Work out the finished part from the listing and answer in its coordinate system (mm). Give positions to 0.01 mm unless a question says otherwise; leave off trailing zeros. Order: outer loops, then holes, each group sorted by start corner. A loop starts at its lowest first (then second) coordinate and runs counter-clockwise, first axis right, second up. Notation, with made-up numbers: M -26,47 L -13,47 A24 ccw -13,66 Z; hole C 61,50 d9. An arc over 180 degrees is marked long. One line per item, written item: value.
Autodesk Inventor part; units mm, degrees
ref_plane "YZ Plane" through (0, 0, 0) normal (1, 0, 0) x (0, 1, 0)
ref_plane "XZ Plane" through (0, 0, 0) normal (0, 1, 0) x (-1, 0, 0)
ref_plane "XY Plane" through (0, 0, 0) normal (0, 0, 1) x (1, 0, 0)
sketch "Sketch1" plane through (0, 0, 0) normal (0, 0, 1) x (1, 0, 0)
  circle A0 centre (0, 0) radius 8.75
  circle A1 centre (0.25, 0) radius 24.8
  circle A2 centre (0.25, 0) radius 4.7
  circle A3 centre (-7.45, 0) radius 1.3
  circle A4 centre (-5.1947, -5.4447) radius 1.3
  circle A5 centre (0.25, -7.7) radius 1.3
  circle A6 centre (5.6947, -5.4447) radius 1.3
  circle A7 centre (7.95, 0) radius 1.3
  circle A8 centre (5.6947, 5.4447) radius 1.3
  circle A9 centre (0.25, 7.7) radius 1.3
  circle A10 centre (-5.1947, 5.4447) radius 1.3
  dimension "d0" = 17.5
  dimension "d1" = 49.6
  dimension "d3" = 9.4
  dimension "d4" = 2.6
  dimension "d7" = 360
extrude "Extrusion1" add sketch "Sketch1" along normal blind 2.5 contours A0 A7 | A0 A7 | A3 | A7 A0 A6 A5 A4 A10 A9 A8 | A8 A0 | A0 A8 | A6 A0 | A0 A6 | A9 A0 | A0 A9 | A5 A0 | A0 A5 | A10 A0 | A0 A10 | A4 A0 | A0 A4
properties part number "BigGearCenterer"
(1) Section A-A, the plane x = 0.25 is taken. Give the vertices of the cut face in (y, z), then the cut area to 3 significant figures.
Findings:
outline: M -9,0 L -4.7,0 L -4.7,2.5 L -9,2.5 Z; M 4.7,0 L 9,0 L 9,2.5 L 4.7,2.5 Z
area: 21.5 mm^2
(2) Determine the mould class of faces 1 (the cylindrical face through (-0.77, 4.59, 1.23)), 2 (the cylindrical face through (8.122, -3.255, 1.232)), 3 (the flat face through (-4, 4, 2.5)), 4 (the cylindrical face through (-3.249, -8.125, 1.232)) for opening direction X: pulls with the +X half, pulls with the -X half, needs draft (parallel to the pull), parting line crosses it, or undercut.
Findings:
face 1: undercut
face 2: pulls with the +X half
face 3: needs draft
face 4: pulls with the -X half
(3) Section D-D, the plane y = 5.5 is taken. Give the vertices of the cut face in (x, z).
Findings:
outline: M -6.81,0 L 6.99,0 L 6.99,2.5 L -6.81,2.5 Z
(4) Given P1, Ø1, axis at x = 6.5, z = 0.5, coming from the +Y side; P2, Ø1, axis at x = -2.5, y = 1.5, coming from the +Z side, each flat-ended and moving along its own axis, determine where each tip first touches the part or whether it passes through.
Findings:
P1: stops at y = 6.71
P2: passes through
(5) Find the intervals of material crossed by probe 1 along Y at (x, z) = (0.25, 1.5); probe 2 along Y at (x, z) = (-2.5, 1.7); probe 3 along X at (y, z) = (2, 0.55), in increasing order. Write a range as from..to.
Findings:
probe 1: y = -9..-4.7, 4.7..9
probe 2: y = -8.39..-3.81, 3.81..8.39
probe 3: x = -8.52..-4, 4.5..8.52
(6) Section B-B, the plane z = 0.6 is taken. Give the vertices of the cut face in (x, y), then the cut area to 3 significant figures.
Findings:
outline: M -6.37,-6 A1.3 ccw -5.69,-6.65 A8.75 ccw -0.54,-8.73 A1.3 ccw 1.1,-8.68 A8.75 ccw 5.58,-6.74 A1.3 ccw 6.98,-5.27 A8.75 ccw 8.68,-1.07 A1.3 ccw 8.68,1.07 A8.75 ccw 6.98,5.27 A1.3 ccw 5.58,6.74 A8.75 ccw 1.1,8.68 A1.3 ccw -0.54,8.73 A8.75 ccw -5.69,6.65 A1.3 ccw -6.37,6 A8.75 ccw Z; hole C 0.25,0 d9.4
area: 174 mm^2
(7) Section C-C, the plane y = -3.25 is taken. Give the vertices of the cut face in (x, z), then the cut area to 3 significant figures.
Findings:
outline: M -8.12,0 L -3.15,0 L -3.15,2.5 L -8.12,2.5 Z; M 3.65,0 L 8.12,0 L 8.12,2.5 L 3.65,2.5 Z
area: 23.6 mm^2
